from build123d import *

# Parameters (mm, degrees)
F1_DEPTH = 20
F3_DEPTH = 4
F4_W     = 33.5
F4_H     = 5
F5_DEPTH = 10.001
F6_DEPTH = 10.001
F7_DEPTH = 10.001


with BuildPart() as f1:
    # F0 (on Front) → F1 (new body)
    with BuildSketch(Plane.XZ):
        with BuildLine():
            Line((30, 51.9615242271), (0, 0))
            Line((0, 0), (130, 0))
            Line((130, 0), (130, 10))
            Line((130, 10), (82.6794919243, 10))
            Line((82.6794919243, 10), (63.2073381993, 21.2422531948))
            ThreePointArc((63.2073381993, 21.2422531948), (62.4652978589, 22.6956144115), (63.4890923627, 23.9663336987))
            Line((63.4890923627, 23.9663336987), (46.168584287, 33.9663336987))
            Line((46.168584287, 33.9663336987), (45.668584287, 33.1003082949))
            ThreePointArc((45.668584287, 33.1003082949), (44.757774749, 32.4014195555), (43.6195461814, 32.5512701892))
            Line((43.6195461814, 32.5512701892), (27.5980762114, 41.8012701892))
            ThreePointArc((27.5980762114, 41.8012701892), (26.8991874719, 42.7120797272), (27.0490381057, 43.8503082949))
            Line((27.0490381057, 43.8503082949), (31.2990381057, 51.2115242271))
            Line((31.2990381057, 51.2115242271), (30, 51.9615242271))
        make_face()
        with BuildLine():
            ThreePointArc((24.5490381057, 36.0560796608), (27.5850698991, 38.3857087923), (31.3791651246, 37.8862066798))
            Line((31.3791651246, 37.8862066798), (94.4019237886, 1.5))
            Line((94.4019237886, 1.5), (27.4019237886, 1.5))
            Line((27.4019237886, 1.5), (14.5543888066, 8.9175277803))
            Line((14.5543888066, 8.9175277803), (10.2990381057, 11.374355653))
            Line((10.2990381057, 11.374355653), (24.5490381057, 36.0560796608))
        make_face(mode=Mode.SUBTRACT)
    extrude(amount=F1_DEPTH)

    # F2 (on face) → F3 (cut)
    with BuildSketch(Plane(origin=(26.25, 0, 45.4663336987), x_dir=(0.8660254038, 0, -0.5), z_dir=(0.5, 0, 0.8660254038))):
        with BuildLine():
            Line((35.949893862, -5.2802399732), (29.1481667175, -5.2802399732))
            ThreePointArc((29.1481667175, -5.2802399732), (24.4296125838, -10.1066845691), (29.3614813401, -14.7149370709))
            Line((29.3614813401, -14.7149370709), (35.7365792394, -14.7149370709))
            ThreePointArc((35.7365792394, -14.7149370709), (40.6684479957, -10.1066845691), (35.949893862, -5.2802399732))
        make_face()
    extrude(amount=-F3_DEPTH, mode=Mode.SUBTRACT)

    # F4 (on face) → F5 (cut, through all)
    with BuildSketch(Plane.XY.offset(10)):
        with Locations((113.25, -2.5)):
            Rectangle(F4_W, F4_H)
    extrude(amount=-F5_DEPTH, mode=Mode.SUBTRACT)

    # F4 (on face) → F6 (cut, through all)
    with BuildSketch(Plane.XY.offset(10)):
        with BuildLine():
            Line((130, -13), (130, -7))
            Line((130, -7), (113, -7))
            ThreePointArc((113, -7), (110, -10), (113, -13))
            Line((113, -13), (130, -13))
        make_face()
    extrude(amount=-F6_DEPTH, mode=Mode.SUBTRACT)

    # F4 (on face) → F7 (cut, through all)
    with BuildSketch(Plane.XY.offset(10)):
        with Locations((113.25, -17.5)):
            Rectangle(F4_W, F4_H)
    extrude(amount=-F7_DEPTH, mode=Mode.SUBTRACT)


solid = f1.part
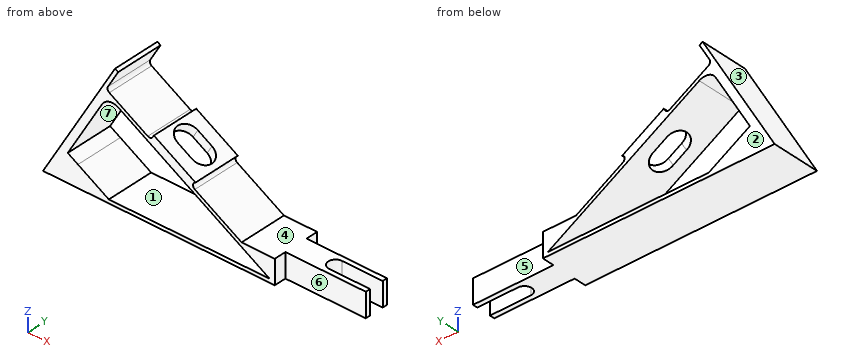
Can you work these out from the model? Positions are in its coordinate system, mm. Face numbers are marked on the shaded views. A direction names the side the tool comes from. Give positions to 0.01 mm unless a question says otherwise; leave off trailing zeros. Order: outer loops, then holes, each group sorted by start corner. A loop starts at its lowest first (then second) coordinate and runs counter-clockwise, first axis right, second up. Notation, with made-up numbers: M 5,52 L 30,52 A23 cw 30,83 Z; hole C -25,74 d6. An arc over 180 degrees is marked long. Use one line per item in the form item = value. Start each with the question number.
Item 1: We'd pull the mould along Z, two halves only. Please class the marked faces 1, 2 and 3: +Z half, -Z half, draft (parallel to the pull), parting line (faces both ways), or undercut.
Item 2: If we section it at A-A (z = 4): Write out the boundary of the cut face in (x, y).
Item 3: If we section it at B-B (y = -16.5): Write out the boundary of the cut face in (x, z).
Item 4: For the marked faces 4, 5, 6 and 7, which set-ups out of +Z, -Z, +X, -X, +Y, -Y let a thin tool reach every point of the face, with its end or its side?
Item 5: If I drill on line 1 along Z through (x, y) = (72, -16); line 2 along Y through (x, z) = (56.5, 25); line 3 along X through (y, z) = (-2.5, 8), over which ranges is the centre line in solid material (lowest first)?
Item 6: If we section it at D-D (y = -10): Write out the boundary of the cut face in (x, z), then the cut area to 3 significant figures.
Item 7: Will these pins go through, and if not, where does the flat tip stop? pin 1 Ø5 at (x, z) = (118, 2.5) entering from -Y; pin 2 Ø5 at (x, z) = (115.5, 4) entering from +Y; pin 3 Ø5 at (y, z) = (-14.5, 34) entering from +X.
Item 8: If we section it at C-C (x = 38): Write out the boundary of the cut face in (y, z), then the cut area to 3 significant figures.
Outcome:
q1.face_1 = undercut
q1.face_2 = draft
q1.face_3 = +Z half
q2.outline = M 2.31,-20 L 23.07,-20 L 23.07,0 L 2.31,0 Z; M 90.07,-20 L 96.5,-20 L 96.5,-15 L 130,-15 L 130,-13 L 113,-13 A3 cw 113,-7 L 130,-7 L 130,-5 L 96.5,-5 L 96.5,0 L 90.07,0 Z
q3.outline = M 0,0 L 96.5,0 L 96.5,10 L 82.68,10 L 63.21,21.24 A1.5 cw 63.49,23.97 L 46.17,33.97 L 45.67,33.1 A1.5 cw 43.62,32.55 L 27.6,41.8 A1.5 cw 27.05,43.85 L 31.3,51.21 L 30,51.96 Z; hole M 10.3,11.37 L 27.4,1.5 L 94.4,1.5 L 31.38,37.89 A5 ccw 24.55,36.06 Z
q4.face_4 = +Z, +X, +Y, -Y
q4.face_5 = +Z, -Z, +X, +Y
q4.face_6 = +Z, -Z, +X, -Y
q4.face_7 = +Y, -Y
q5.line_1 = 0 to 1.5, 14.43 to 16.17
q5.line_2 = -20 to -14.7, -5.3 to 0
q5.line_3 = 4.62 to 16.14, 83.14 to 96.5
q6.outline = M 0,0 L 110,0 L 110,10 L 82.68,10 L 63.21,21.24 A1.5 cw 63.49,23.97 L 61.47,25.13 L 59.47,21.67 L 94.4,1.5 L 27.4,1.5 L 10.3,11.37 L 24.55,36.06 A5 cw 31.38,37.89 L 45.41,29.79 L 47.41,33.25 L 46.17,33.97 L 45.67,33.1 A1.5 cw 43.62,32.55 L 27.6,41.8 A1.5 cw 27.05,43.85 L 31.3,51.21 L 30,51.96 Z
q6.area = 724 mm2
q7.pin_1 = -15
q7.pin_2 = -5
q7.pin_3 = 50.44
q8.outline = M -20,0 L 0,0 L 0,1.5 L -20,1.5 Z; M -20,34.06 L 0,34.06 L 0,35.8 L -20,35.8 Z
q8.area = 64.6 mm2
